Design review of the part built by this model. Coordinates are the model's own, in mm. A direction names the side the tool comes from. Give positions to 0.01 mm unless a question says otherwise; leave off trailing zeros. Use CSV: the item, a comma, the result in double quotes.
```python
from build123d import *

# Parameters (mm, degrees)
RESSALTO_EXTRUS_O1_DEPTH   = 285
CORTE_EXTRUS_O1_DEPTH      = 1
CORTE_EXTRUS_O1_DEPTH_BACK = 286
ESBO_O4_R                  = 1.25
CORTE_EXTRUS_O3_DEPTH      = 10
ESBO_O7_R                  = 1.65
ESBO_O7_R_2                = 1.25
CORTE_EXTRUS_O5_DEPTH      = 4
ESBO_O13_R                 = 1.75
CORTE_EXTRUS_O8_DEPTH      = 3.5
CORTE_EXTRUS_O8_DEPTH_BACK = 28.5
ESBO_O14_R                 = 1.25
CORTE_EXTRUS_O9_DEPTH      = 5


with BuildPart() as part:
    # Esboço1 → Ressalto-extrusão1 (new body)
    with BuildSketch(Plane.XY):
        with BuildLine():
            Line((0, 0), (-113, 0))
            Line((-113, 0), (-113, 30))
            Line((-113, 30), (-111, 30))
            Line((-111, 30), (-111, 6))
            Line((-111, 6), (-107.3, 6))
            Line((-107.3, 6), (-106.5, 29))
            ThreePointArc((-106.5, 29), (-105.5, 30), (-104.5, 29))
            Line((-104.5, 29), (-104, 6))
            Line((-104, 6), (-100.3, 6))
            Line((-100.3, 6), (-99.5, 29))
            ThreePointArc((-99.5, 29), (-98.5, 30), (-97.5, 29))
            Line((-97.5, 29), (-97, 6))
            Line((-97, 6), (-93.3, 6))
            Line((-93.3, 6), (-92.5, 29))
            ThreePointArc((-92.5, 29), (-91.5, 30), (-90.5, 29))
            Line((-90.5, 29), (-90, 6))
            Line((-90, 6), (-86.3, 6))
            Line((-86.3, 6), (-85.5, 29))
            ThreePointArc((-85.5, 29), (-84.5, 30), (-83.5, 29))
            Line((-83.5, 29), (-83, 6))
            Line((-83, 6), (-79.3, 6))
            Line((-79.3, 6), (-78.5, 29))
            ThreePointArc((-78.5, 29), (-77.5, 30), (-76.5, 29))
            Line((-76.5, 29), (-76, 6))
            Line((-76, 6), (-72.3, 6))
            Line((-72.3, 6), (-71.5, 29))
            ThreePointArc((-71.5, 29), (-70.5, 30), (-69.5, 29))
            Line((-69.5, 29), (-69, 6))
            Line((-69, 6), (-65.3, 6))
            Line((-65.3, 6), (-64.5, 29))
            ThreePointArc((-64.5, 29), (-63.5, 30), (-62.5, 29))
            Line((-62.5, 29), (-62, 6))
            Line((-62, 6), (-58.3, 6))
            Line((-58.3, 6), (-57.5, 29))
            ThreePointArc((-57.5, 29), (-56.5, 30), (-55.5, 29))
            Line((-55.5, 29), (-54.7, 6))
            Line((-54.7, 6), (-51, 6))
            Line((-51, 6), (-50.5, 29))
            ThreePointArc((-50.5, 29), (-49.5, 30), (-48.5, 29))
            Line((-48.5, 29), (-47.7, 6))
            Line((-47.7, 6), (-44, 6))
            Line((-44, 6), (-43.5, 29))
            ThreePointArc((-43.5, 29), (-42.5, 30), (-41.5, 29))
            Line((-41.5, 29), (-40.7, 6))
            Line((-40.7, 6), (-37, 6))
            Line((-37, 6), (-36.5, 29))
            ThreePointArc((-36.5, 29), (-35.5, 30), (-34.5, 29))
            Line((-34.5, 29), (-33.7, 6))
            Line((-33.7, 6), (-30, 6))
            Line((-30, 6), (-29.5, 29))
            ThreePointArc((-29.5, 29), (-28.5, 30), (-27.5, 29))
            Line((-27.5, 29), (-26.7, 6))
            Line((-26.7, 6), (-23, 6))
            Line((-23, 6), (-22.5, 29))
            ThreePointArc((-22.5, 29), (-21.5, 30), (-20.5, 29))
            Line((-20.5, 29), (-19.7, 6))
            Line((-19.7, 6), (-16, 6))
            Line((-16, 6), (-15.5, 29))
            ThreePointArc((-15.5, 29), (-14.5, 30), (-13.5, 29))
            Line((-13.5, 29), (-12.7, 6))
            Line((-12.7, 6), (-9, 6))
            Line((-9, 6), (-8.5, 29))
            ThreePointArc((-8.5, 29), (-7.5, 30), (-6.5, 29))
            Line((-6.5, 29), (-5.7, 6))
            Line((-5.7, 6), (-2, 6))
            Line((-2, 6), (-2, 30))
            Line((-2, 30), (0, 30))
            Line((0, 30), (0, 0))
        make_face()
    extrude(amount=RESSALTO_EXTRUS_O1_DEPTH)

    # Esboço2 → Corte-extrusão1 (cut, two sides)
    with BuildSketch(Plane.XY.offset(285)) as corte_extrus_o1_sk:
        Polygon((-102.890485004, 6), (-108.234061138, 6), (-108.234061138, 2.5), (-102.553847577, 2.5), (-102.553847577, 0), (-107.964469124, -3.436706701), (-125.556799279, -3.436706701), (-125.556799279, 31.540588642), (-102.890485004, 31.540588642), align=None)
        Polygon((-8.281088913, 1.25), (-10.446152423, 0), (0, 0), (0, 38.558769493), (-11.416815759, 38.558769493), (-11.416815759, 6.681238216), align=None)
    extrude(amount=CORTE_EXTRUS_O1_DEPTH, mode=Mode.SUBTRACT)
    extrude(corte_extrus_o1_sk.sketch, amount=-CORTE_EXTRUS_O1_DEPTH_BACK, mode=Mode.SUBTRACT)

    # Esboço4 → Corte-extrusão3 (cut)
    with BuildSketch(Plane.XY.offset(285)):
        with Locations((-26.5, 3.234792224)):
            Circle(ESBO_O4_R)
        with Locations((-86.5, 3.234792224)):
            Circle(ESBO_O4_R)
    extrude(amount=-CORTE_EXTRUS_O3_DEPTH, mode=Mode.SUBTRACT)

    # Esboço7 → Corte-extrusão5 (cut)
    with BuildSketch(Plane(origin=(0, 0, 0), x_dir=(-1, 0, 0), z_dir=(0, -1, 0))):
        with Locations((95, -28.5)):
            Circle(ESBO_O7_R)
        with Locations((71.949, -28.592)):
            Circle(ESBO_O7_R_2)
        with Locations((72.33, -10.685)):
            Circle(ESBO_O7_R_2)
        with Locations((30.928, -51.5)):
            Circle(ESBO_O7_R_2)
        with Locations((24, -15)):
            Circle(ESBO_O7_R)
        with Locations((34.738, -79.011)):
            Circle(ESBO_O7_R_2)
        with Locations((18.355, -144.416)):
            Circle(ESBO_O7_R)
        with Locations((20, -249)):
            Circle(ESBO_O7_R)
        with Locations((35.246, -237)):
            Circle(ESBO_O7_R_2)
        with Locations((93, -249)):
            Circle(ESBO_O7_R)
        with Locations((78.807, -182.77)):
            Circle(ESBO_O7_R_2)
        with Locations((82.363, -100.093)):
            Circle(ESBO_O7_R_2)
        with Locations((29.404, -176.293)):
            Circle(ESBO_O7_R_2)
        with Locations((38.999998474, -219.999999573)):
            Circle(ESBO_O7_R_2)
        with Locations((38.999998474, -199.999999573)):
            Circle(ESBO_O7_R_2)
        with Locations((38.999998474, -179.999999573)):
            Circle(ESBO_O7_R_2)
        with Locations((38.999998474, -159.999999573)):
            Circle(ESBO_O7_R_2)
        with Locations((73.999998474, -129.999991943)):
            Circle(ESBO_O7_R_2)
        with Locations((73.999998474, -110.000007202)):
            Circle(ESBO_O7_R_2)
        with Locations((73.999998474, -90.000007202)):
            Circle(ESBO_O7_R_2)
        with Locations((73.999998474, -69.999991943)):
            Circle(ESBO_O7_R_2)
        with Locations((92.737766412, -168.347796909)):
            Circle(ESBO_O7_R_2)
        with Locations((94.207008215, -195.602168929)):
            Circle(ESBO_O7_R_2)
        with Locations((89.504149751, -51.5)):
            Circle(ESBO_O7_R_2)
        with Locations((49.75, -279)):
            Circle(ESBO_O7_R_2)
        with Locations((63.25, -279)):
            Circle(ESBO_O7_R_2)
    extrude(amount=-CORTE_EXTRUS_O5_DEPTH, mode=Mode.SUBTRACT)

    # Esboço13 → Corte-extrusão8 (cut, two sides)
    with BuildSketch(Plane.XZ.offset(-2.5)) as corte_extrus_o8_sk:
        with Locations((-105.393954358, 275)):
            Circle(ESBO_O13_R)
        with Locations((-105.393954358, 222)):
            Circle(ESBO_O13_R)
        with Locations((-105.393954358, 169)):
            Circle(ESBO_O13_R)
        with Locations((-105.393954358, 63)):
            Circle(ESBO_O13_R)
        with Locations((-105.393954358, 10)):
            Circle(ESBO_O13_R)
        with Locations((-105.393954358, 116)):
            Circle(ESBO_O13_R)
    extrude(amount=CORTE_EXTRUS_O8_DEPTH, mode=Mode.SUBTRACT)
    extrude(corte_extrus_o8_sk.sketch, amount=-CORTE_EXTRUS_O8_DEPTH_BACK, mode=Mode.SUBTRACT)

    # Esboço14 → Corte-extrusão9 (cut)
    with BuildSketch(Plane(origin=(-5.669550808, -3.273316685, 0), x_dir=(0, 0, -1), z_dir=(0.866025404, 0.5, 0))):
        with Locations((-275, 8.063182992)):
            Circle(ESBO_O14_R)
        with Locations((-222, 8.063182992)):
            Circle(ESBO_O14_R)
        with Locations((-169, 8.063182992)):
            Circle(ESBO_O14_R)
        with Locations((-116, 8.063182992)):
            Circle(ESBO_O14_R)
        with Locations((-63, 8.063182992)):
            Circle(ESBO_O14_R)
        with Locations((-10, 8.063182992)):
            Circle(ESBO_O14_R)
    extrude(amount=-CORTE_EXTRUS_O9_DEPTH, mode=Mode.SUBTRACT)


solid = part.part
```
(1) Mouldability with a two-part tool opening along Y and no side actions: class faces 3 (the face through (-11.86, 2.52, 11.25)), 4 (the face through (-57.6, 11.9, 285)), 5 (the face through (-9.671, 3.658, 144.495)) as +Y half, -Y half, draft (parallel to the pull), parting line (faces both ways), or undercut.
Established:
face 3,"undercut"
face 4,"draft"
face 5,"+Y half"
(2) Clearance check with flat-ended pins moving along their axes: pin 1 (2 mm diameter, centred on x = -73.5, z = 90.5, fed in from -Y); pin 2 (1.6 mm diameter, centred on x = -24, z = 14.5, fed in from -Y); pin 3 (4.5 mm diameter, centred on x = -105.39, z = 169, fed in from -Y); pin 4 (2 mm diameter, centred on x = -74, z = 130, fed in from +Y). State where each tip first meets the part, or that it passes through.
Established:
pin 1,"stops at y = 0"
pin 2,"stops at y = 4"
pin 3,"stops at y = 2.5"
pin 4,"stops at y = 6"
(3) Take a section at A-A (y = 9.5). State how many separate pieces and enclosed holes the cut face has, then the cut area to 3 significant figures.
Established:
separate pieces,"13"
enclosed holes,"0"
area,"11,600 mm2"
(4) For line 1 along Z through (x, y) = (-82.5, 1.5); line 2 along Y through (x, z) = (-101.5, 234.5); line 3 along Y through (x, z) = (-26.5, 278.75), list the stretches that pass through material, from the lowest coordinate up. Write a range as [from, to].
Established:
line 1,"z = [0, 98.85], [101.34, 285]"
line 2,"y = [0, 6]"
line 3,"y = [0, 1.98], [4.48, 6]"
(5) Tool access review of faces 1 (the face through (-12.024, 2.802, 114.808)), 2 (the face through (-104, 6, 141)): name each direction out of +Z, -Z, +X, -X, +Y, -Y from which nothing blocks a thin tool from reaching the whole face with its end or side.
Established:
face 1,"none"
face 2,"+Z, -Z, -X, +Y"
